```python
from build123d import *

# Parameters (mm, degrees)
SKETCH_1_W          = 65
SKETCH_1_H          = 20
EXTRUDE_1_DEPTH     = 10
CUT_EXTRUDE_1_DEPTH = 10
FILLET_1_R          = 3


with BuildPart() as part:
    # 草图1 → 凸台-拉伸1 (new body)
    with BuildSketch(Plane(origin=(0, 0, 0), x_dir=(1, 0, 0), z_dir=(0, 1, 0))):
        Rectangle(SKETCH_1_W, SKETCH_1_H)
    extrude(amount=EXTRUDE_1_DEPTH)

    # 草图2 → 切除-拉伸1 (cut)
    with BuildSketch(Plane(origin=(0, 10, 0), x_dir=(1, 0, 0), z_dir=(0, 1, 0))):
        with BuildLine():
            Line((-27.375, 1.6), (-19.5, 1.6))
            ThreePointArc((-19.5, 1.6), (-17.9, 0), (-19.5, -1.6))
            Line((-19.5, -1.6), (-27.375, -1.6))
            ThreePointArc((-27.375, -1.6), (-28.975, 0), (-27.375, 1.6))
        make_face()
        with BuildLine():
            Line((27.375, 1.6), (19.5, 1.6))
            ThreePointArc((19.5, 1.6), (17.9, 0), (19.5, -1.6))
            Line((19.5, -1.6), (27.375, -1.6))
            ThreePointArc((27.375, -1.6), (28.975, 0), (27.375, 1.6))
        make_face()
    extrude(amount=-CUT_EXTRUDE_1_DEPTH, mode=Mode.SUBTRACT)

    # 圆角1
    fillet_1_edges = [part.edges().sort_by_distance(p)[0] for p in [
        (32.5, 5, 10),
        (-32.5, 5, 10),
        (-32.5, 5, -10),
        (32.5, 5, -10),
    ]]
    fillet(fillet_1_edges, radius=FILLET_1_R)


solid = part.part
```
Verification items for the finished model (mm, model axes). A direction names the side the tool comes from. Give positions to 0.01 mm unless a question says otherwise; leave off trailing zeros. Order: outer loops, then holes, each group sorted by start corner. A loop starts at its lowest first (then second) coordinate and runs counter-clockwise, first axis right, second up. Notation, with made-up numbers: M 62.5,-4 L 93.5,-4 A13 cw 93.5,20 Z; hole C 30.25,-17.75 d4. An arc over 180 degrees is marked long. Answer in a Markdown table with one row per item. Add a question column.
Item 1: Gauge pin test, flat end, axial feed: pin 1 (1.5 mm diameter, centred on x = 17, z = 4, fed in from -Y). Record the tip position at first contact, or that the pin passes through.
Item 2: Mould release check, pull along Z, two halves, no side actions. Record for faces 1 (the flat face through (-32.5, 5, 0)), 2 (the cylindrical face through (-31.64, 5.07, 9.1)), 3 (the flat face through (-23, 5, -1.6)), 4 (the cylindrical face through (-28.975, 5.07, 0.035)): released by +Z, released by -Z, zero draft, split by the parting line, or undercut.
Item 3: Scan lines: probe 1 along Z at (x, y) = (-25.5, 1.25); probe 2 along X at (y, z) = (6.25, -1); probe 3 along Z at (x, y) = (-28.5, 9.25). Record each from-to range of solid material in increasing order. Write a range as from..to.
Item 4: Tool access check on faces 5 (the flat face through (23, 5, 1.6)), 6 (the flat face through (0, 5, 10)). Record the directions out of +Z, -Z, +X, -X, +Y, -Y that give a thin tool (end or side, any length) a straight path to the whole face; none if there is none.
Item 5: Section check B-B, the plane z = 0. Enter the section's corners in (x, y) (3 decimals), and give its area (4 significant figures).
Item 6: Section check A-A, the plane x = 23. Enter the section's corners in (y, z), and give its area (3 significant figures).
Item 7: Section check C-C, the plane y = 9.25. Enter the section's corners in (x, z) (3 decimals), and give its area (3 significant figures).
Filled sheet:
| question | item | result |
|---|---|---|
| 1 | pin 1 | stops at y = 0 |
| 2 | face 1 | zero draft |
| 2 | face 2 | released by +Z |
| 2 | face 3 | undercut |
| 2 | face 4 | undercut |
| 3 | probe 1 | z = -10..-1.6, 1.6..10 |
| 3 | probe 2 | x = -32.5..-28.62, -18.25..18.25, 28.62..32.5 |
| 3 | probe 3 | z = -10..-1.14, 1.14..10 |
| 4 | face 5 | +Y, -Y |
| 4 | face 6 | +Z, +X, -X, +Y, -Y |
| 5 | outline | M -32.5,0 L -28.975,0 L -28.975,10 L -32.5,10 Z; M -17.9,0 L 17.9,0 L 17.9,10 L -17.9,10 Z; M 28.975,0 L 32.5,0 L 32.5,10 L 28.975,10 Z |
| 5 | area | 428.5 mm^2 |
| 6 | outline | M 0,-10 L 10,-10 L 10,-1.6 L 0,-1.6 Z; M 0,1.6 L 10,1.6 L 10,10 L 0,10 Z |
| 6 | area | 168 mm^2 |
| 7 | outline | M -32.5,-7 A3 ccw -29.5,-10 L 29.5,-10 A3 ccw 32.5,-7 L 32.5,7 A3 ccw 29.5,10 L -29.5,10 A3 ccw -32.5,7 Z; hole M -27.375,-1.6 L -19.5,-1.6 A1.6 ccw -19.5,1.6 L -27.375,1.6 A1.6 ccw Z; hole M 19.5,-1.6 L 27.375,-1.6 A1.6 ccw 27.375,1.6 L 19.5,1.6 A1.6 ccw Z |
| 7 | area | 1,230 mm^2 |
